Model file for the job. Use its own axes, mm. A direction names the side the tool comes from. Round coordinates to 2 decimals unless told otherwise and drop trailing zeros. Order: outer loops, then holes, each group sorted by start corner. A loop starts at its lowest first (then second) coordinate and runs counter-clockwise, first axis right, second up. Notation, with made-up numbers: (-2.5, -11) -> (21.5, -11) arc R28 cw to (21.5, 8) -> close; hole circle Ø2 at (44, 46). An arc over 180 degrees is marked (long way). Put each result on its own line as item: value. Start each with the question number.
Q1. Pull direction X, two halves, no side cores. Call faces 1 (the face through (7, -10.75, 0)), 2 (the face through (10.45, -9, 0)), 3 (the face through (4.53, 2.35, 0.02)), 4 (the face through (5.65, -5, 0)): released by +X, released by -X, zero draft, split by the parting line, or undercut.
Q2. 3-axis set-ups, long thin cutter, end or side, ignore diameter. For faces 5 (the face through (3.45, -5, 0)), 6 (the face through (0, -10.75, 0)): which of +Z, -Z, +X, -X, +Y, -Y reach the whole face in a straight line?
Q3. Cut at C-C, the plane y = -9.5. List the corners of the cut face in (x, z), and give its area (3 significant figures).
Q4. Cut at A-A, the plane y = 1. List the corners of the cut face in (x, z), and give its area (3 significant figures).
Q5. Flat gauge pins, fed straight in: P1, Ø1, axis at y = -5, z = 0, coming from the -X side; P2, Ø0.6, axis at x = 8.5, z = 0, coming from the +Y side; P3, Ø1, axis at y = 7.5, z = 0, coming from the +X side. Where does each tip first touch, or does it go through?
Q6. Cut at B-B, the plane x = -4.55. List the corners of the cut face in (y, z), and give its area (3 significant figures).
Q7. Cut at D-D, the plane z = -0.8. List the corners of the cut face in (x, y).
Q8. Probe L1, parallel to X at y = -0.5, z = -0.5; L2, parallel to X at y = 1.75, z = 0.85; L3, parallel to X at y = 7, z = -0.1. List the from-to ranges inside material, lowest first.
from build123d import *

# Parameters (mm, degrees)
F1_DEPTH = 1.45
F0_W     = 2.3
F0_H     = 1.25
F4_SIZE2 = 1.2
F4_SIZE  = 2.5
F0_W_2   = 0.5
F0_H_2   = 1.5
F5_DEPTH = 0.25
F6_DEPTH = 0.25


with BuildPart() as f1:
    # F0 (on Top) → F1 (new body, symmetric)
    with BuildSketch(Plane.XY):
        with BuildLine():
            Line((8.15, -6.74), (8.15, 10.75))
            Line((8.15, 10.75), (-8.15, 10.75))
            Line((-8.15, 10.75), (-8.15, -6.74))
            Line((-8.15, -6.74), (-8.15, -8.24))
            Line((-8.15, -8.24), (-8.15, -8.25))
            Line((-8.15, -8.25), (-8.15, -9.5))
            Line((-8.15, -9.5), (-8.15, -10.75))
            Line((-8.15, -10.75), (-5.65, -10.75))
            Line((-5.65, -10.75), (-5.65, 1.25))
            ThreePointArc((-5.65, 1.25), (-4.55, 2.35), (-3.45, 1.25))
            Line((-3.45, 1.25), (-3.45, -10.75))
            Line((-3.45, -10.75), (3.45, -10.75))
            Line((3.45, -10.75), (3.45, 1.25))
            ThreePointArc((3.45, 1.25), (4.55, 2.35), (5.65, 1.25))
            Line((5.65, 1.25), (5.65, -10.75))
            Line((5.65, -10.75), (8.15, -10.75))
            Line((8.15, -10.75), (8.15, -9.5))
            Line((8.15, -9.5), (8.15, -8.25))
            Line((8.15, -8.25), (8.15, -8.24))
            Line((8.15, -8.24), (8.15, -6.74))
        make_face()
    extrude(amount=F1_DEPTH, both=True)

    # F0 (on Top) → F2 (revolve)
    with BuildSketch(Plane.XY):
        with Locations((9.3, -10.125)):
            Rectangle(F0_W, F0_H)
    revolve(axis=Axis((9.3, -9.5, 0), (1, 0, 0)))

    # F0 (on Top) → F3 (revolve)
    with BuildSketch(Plane.XY):
        with Locations((-9.3, -10.125)):
            Rectangle(F0_W, F0_H)
    revolve(axis=Axis((-9.3, -9.5, 0), (-1, 0, 0)))

    # F4
    f4_edges = [f1.edges().sort_by_distance(p)[0] for p in [
        (0, 10.75, 1.45),
    ]]
    chamfer(f4_edges, length=F4_SIZE, length2=F4_SIZE2)

    # F0 (on Top) → F5 (join, symmetric)
    with BuildSketch(Plane.XY):
        with Locations((8.4, -7.49)):
            Rectangle(F0_W_2, F0_H_2)
    extrude(amount=F5_DEPTH, both=True)

    # F0 (on Top) → F6 (join, symmetric)
    with BuildSketch(Plane.XY):
        with Locations((-8.4, -7.49)):
            Rectangle(F0_W_2, F0_H_2)
    extrude(amount=F6_DEPTH, both=True)


solid = f1.part
Ans:
1. face 1: zero draft
1. face 2: released by +X
1. face 3: undercut
1. face 4: undercut
2. face 5: +Z, -Z, -Y
2. face 6: +Z, -Z, +X, -X, -Y
3. outline: (-10.45, -1.25) -> (-8.15, -1.25) -> (-8.15, -1.45) -> (-5.65, -1.45) -> (-5.65, 1.45) -> (-8.15, 1.45) -> (-8.15, 1.25) -> (-10.45, 1.25) -> close; (-3.45, -1.45) -> (3.45, -1.45) -> (3.45, 1.45) -> (-3.45, 1.45) -> close; (5.65, -1.45) -> (8.15, -1.45) -> (8.15, -1.25) -> (10.45, -1.25) -> (10.45, 1.25) -> (8.15, 1.25) -> (8.15, 1.45) -> (5.65, 1.45) -> close
3. area: 46.0 mm^2
4. outline: (-8.15, -1.45) -> (-5.65, -1.45) -> (-5.65, 1.45) -> (-8.15, 1.45) -> close; (-3.45, -1.45) -> (3.45, -1.45) -> (3.45, 1.45) -> (-3.45, 1.45) -> close; (5.65, -1.45) -> (8.15, -1.45) -> (8.15, 1.45) -> (5.65, 1.45) -> close
4. area: 34.5 mm^2
5. P1: stops at x = -8.15
5. P2: stops at y = -6.74
5. P3: stops at x = 8.15
6. outline: (2.35, -1.45) -> (10.75, -1.45) -> (10.75, -1.05) -> (9.55, 1.45) -> (2.35, 1.45) -> close
6. area: 22.9 mm^2
7. outline: (-10.45, -10.46) -> (-8.15, -10.46) -> (-8.15, -10.75) -> (-5.65, -10.75) -> (-5.65, 1.25) arc R1.1 cw to (-3.45, 1.25) -> (-3.45, -10.75) -> (3.45, -10.75) -> (3.45, 1.25) arc R1.1 cw to (5.65, 1.25) -> (5.65, -10.75) -> (8.15, -10.75) -> (8.15, -10.46) -> (10.45, -10.46) -> (10.45, -8.54) -> (8.15, -8.54) -> (8.15, 10.63) -> (-8.15, 10.63) -> (-8.15, -8.54) -> (-10.45, -8.54) -> close
8. L1: x = -8.15 to -5.65, -3.45 to 3.45, 5.65 to 8.15
8. L2: x = -8.15 to -5.53, -3.57 to 3.57, 5.53 to 8.15
8. L3: x = -8.15 to 8.15
